Autodesk Inventor part; units mm, degrees
ref_plane "YZ Plane" through (0, 0, 0) normal (1, 0, 0) x (0, 1, 0)
ref_plane "XZ Plane" through (0, 0, 0) normal (0, 1, 0) x (-1, 0, 0)
ref_plane "XY Plane" through (0, 0, 0) normal (0, 0, 1) x (1, 0, 0)
sketch "Esboço1" plane through (0, 0, 0) normal (0, 0, 1) x (1, 0, 0)
  circle A0 centre (28.2, 9.3) radius 5.5
  line L0 (-31.3, -7.5) -> (33.7, -7.5) construction
  line L1 (33.7, -7.5) -> (33.7, 14.8) construction
  line L2 (33.7, 14.8) -> (-31.3, 14.8) construction
  line L3 (-31.3, 14.8) -> (-31.3, -7.5) construction
  circle A1 centre (10.85, -0.05) radius 5.5
  line L4 (-14.7338, -7.5) -> (-8.5113, -1.2775)
  line L5 (-31.3, -7.5) -> (-14.7338, -7.5)
  line L6 (-8.5113, -1.2775) -> (5.4887, -1.2775)
  line L7 (-31.3, -7.5) -> (-31.3, 0.8)
  line L8 (-31.3, 0.8) -> (-1.3563, 8.8234)
  line L9 (-1.3563, 8.8234) -> (3.6437, 8.8234)
  line L10 (3.6437, 8.8234) -> (26.4006, 14.4973)
  line L11 (14.415, 4.1381) -> (14.415, 6.5881)
  line L12 (14.415, 6.5881) -> (23.415, 6.5881)
  line L13 (-26.4266, -1) -> (-26.4266, -4.5)
  line L14 (-26.4266, -4.5) -> (-15.9765, -4.5)
  line L15 (-26.4266, -1) -> (-1.3377, 5.7225)
  line L16 (-15.9765, -4.5) -> (-9.7539, 1.7225)
  line L17 (-9.7539, 1.7225) -> (1.1623, 1.7225)
  line L18 (1.1623, 1.7225) -> (1.1623, 5.7225)
  line L19 (1.1623, 5.7225) -> (-1.3377, 5.7225)
  point P0 (0, 0)
  dimension "d4" = 11
  dimension "d5" = 28.2
  dimension "d6" = 9.3
  dimension "d7" = 65
  dimension "d8" = 22.3
  dimension "d9" = 65
  dimension "d10" = 9.35
  dimension "d11" = 17.35
  dimension "d12" = 8.8
  dimension "d14" = 135
  dimension "d15" = 14
  dimension "d16" = 8.3
  dimension "d17" = 31
  dimension "d18" = 105
  dimension "d19" = 5
  dimension "d20" = 14
  dimension "d21" = 2.45
  dimension "d22" = 9
  dimension "d23" = 3
  dimension "d24" = 3
  dimension "d25" = 3.5
  dimension "d26" = 3
  dimension "d27" = 3
  dimension "d28" = 4
  dimension "d29" = 2.5
extrude "Extrusão1" add sketch "Esboço1" along normal blind 2.2 contours A0 L12 L11 A1 L6 L4 L5 L7 L8 L9 L10
extrude "Extrusão2" add sketch "Esboço1" against normal blind 6.6 contours A1
extrude "Extrusão3" add sketch "Esboço1" along normal blind 2.2 contours A0
sketch "Esboço2" plane through (0, 0, 0) normal (0, 0, 1) x (1, 0, 0)
  arc A0 (5.4887, -1.2775) -> (14.415, 4.1381) centre (10.85, -0.05) ccw
  point P0 (0, 0)
hole "Furo1" at (10.85, -0.05, 0) direction (0, 0, -1) diameter 3.5 end through all
sketch "Esboço3" plane through (0, 0, 2.2) normal (0, 0, 1) x (1, 0, 0)
  arc A0 (23.415, 6.5881) -> (26.4006, 14.4973) centre (28.2, 9.3) ccw
  point P0 (0, 0)
hole "Furo2" at (28.2, 9.3, 2.2) direction (0, 0, -1) diameter 3.5 end through all countersink diameter 7 countersink angle 90
pattern_linear "Padrão retangular3" count 2 spacing 8.8 along (0, 0, -1) of "Extrusão1", "Extrusão3"
sketch "Esboço6" plane through (-14.7338, -7.5, -8.8) normal (0, 0, -1) x (-1, 0, 0)
  circle A0 centre (-42.9338, 16.8) radius 3.5
  line L0 (-41.1838, 13.7689) -> (-44.6838, 13.7689)
  line L1 (-44.6838, 13.7689) -> (-46.4338, 16.8)
  line L2 (-46.4338, 16.8) -> (-44.6838, 19.8311)
  line L3 (-44.6838, 19.8311) -> (-41.1838, 19.8311)
  line L4 (-41.1838, 19.8311) -> (-39.4338, 16.8)
  line L5 (-39.4338, 16.8) -> (-41.1838, 13.7689)
  point P0 (-14.7338, 7.5)
  point P1 (-42.9338, 16.8)
extrude "Extrusão6" cut sketch "Esboço6" along normal mid plane 4.4 contours L5 L0 L1 L2 L3 L4
sketch "Esboço4" plane through (0, 0, 0) normal (0, 0, -1) x (-1, 0, 0)
  line L0 (-26.4006, 14.4973) -> (-3.6437, 8.8234)
  line L1 (-26.4006, 14.4973) -> (-3.6437, 8.8234)
  line L2 (1.3563, 8.8234) -> (31.3, 0.8)
  line L3 (-3.6437, 8.8234) -> (1.3563, 8.8234)
  line L4 (1.3563, 8.8234) -> (31.3, 0.8)
  line L5 (31.3, 0.8) -> (31.3, -7.5)
  line L6 (31.3, -7.5) -> (14.7338, -7.5)
  line L7 (31.3, -7.5) -> (14.7338, -7.5)
  line L8 (14.7338, -7.5) -> (8.5113, -1.2775)
  line L9 (15.9765, -4.5) -> (9.7539, 1.7225)
  line L10 (8.5113, -1.2775) -> (-5.4887, -1.2775)
  arc A0 (-5.4887, -1.2775) -> (-14.415, 4.1381) centre (-10.85, -0.05) ccw
  arc A1 (-14.415, 4.1381) -> (-5.4887, -1.2775) centre (-10.85, -0.05) ccw
  line L11 (-14.415, 4.1381) -> (-14.415, 6.5881)
  line L12 (-14.415, 4.1381) -> (-14.415, 6.5881)
  line L13 (-14.415, 6.5881) -> (-23.415, 6.5881)
  line L14 (-14.415, 6.5881) -> (-23.415, 6.5881)
  arc A2 (-26.4006, 14.4973) -> (-23.415, 6.5881) centre (-28.2, 9.3) ccw construction
  arc A3 (-26.4006, 14.4973) -> (-23.415, 6.5881) centre (-28.2, 9.3) ccw
  arc A4 (-23.415, 6.5881) -> (-26.4006, 14.4973) centre (-28.2, 9.3) ccw
  line L15 (-1.1623, 5.7225) -> (1.3377, 5.7225)
  line L16 (-1.1623, 5.7225) -> (1.3377, 5.7225)
  line L17 (26.4266, -1) -> (1.3377, 5.7225)
  line L18 (1.3377, 5.7225) -> (26.4266, -1)
  line L19 (26.4266, -1) -> (26.4266, -4.5)
  line L20 (15.9765, -4.5) -> (26.4266, -4.5)
  line L21 (26.4266, -4.5) -> (15.9765, -4.5)
  line L22 (15.9765, -4.5) -> (9.7539, 1.7225)
  line L23 (9.7539, 1.7225) -> (-1.1623, 1.7225)
  line L24 (-1.1623, 1.7225) -> (-1.1623, 5.7225)
  point P0 (0, 0)
  point P1 (-5.4887, -1.2775)
extrude "Extrusão7" add sketch "Esboço4" along normal blind 6.6 contours L0 L3 L2 L5 L6 L8 L10 A0 L11 L13 A4
properties part number "Pinza_0002_001" material "Borracha"
Check sheet for the modelled part. Datum: model origin and axes. Units: mm. A direction names the side the tool comes from. Round coordinates to 2 decimals unless told otherwise and drop trailing zeros. Order: outer loops, then holes, each group sorted by start corner. A loop starts at its lowest first (then second) coordinate and runs counter-clockwise, first axis right, second up.
(1) Draft check along X on faces 6 (the flat face through (25.56, 7.81, -7.68)), 7 (the flat face through (1, 8.823, -3)), 8 (the flat face through (-16.119, 4.868, -3.223)), 9 (the flat face through (25.59, 10.84, -7.68)). Enter one of: pulls with the +X half, pulls with the -X half, needs draft (parallel to the pull), parting line crosses it, or undercut.
(2) Cross-section at D-D, the plane z = -5. State how many separate pieces and enclosed holes the cut face has, and give its area (3 significant figures).
(3) Access from +Z, -Z, +X, -X, +Y, -Y to the whole of each face (thin tool, end or side, straight path). Record for faces 1 (the flat face through (0, 5.722, -3)), 2 (the flat face through (1, 6, -8.8)), 3 (the flat face through (-31.3, -3, -3)), 4 (the cylindrical face through (7.915, 4.602, 1.085)), 5 (the flat face through (30.84, 10.79, -7.68)).
(4) Go/stop test with flat-tipped pins: P1, Ø4, axis at y = -3, z = -3.5, coming from the +X side; P2, Ø0.7, axis at x = 28, z = -7.5, coming from the -Y side; P3, Ø2.5, axis at x = 1, z = -1.5, coming from the +Y side; P4, Ø12, axis at x = 8.5, y = 0.5, coming from the +Z side. Record where each tip stops, or that it passes through.
(5) Cross-section at B-B, the plane x = -24. Enter the section's corners in (y, z), and give its area (3 significant figures).
(6) Cross-section at A-A, the plane x = 28.2. Enter the section's corners in (y, z).
(7) Cross-section at C-C, the plane y = -3.25. Enter the section's corners in (x, z).
(8) Scan lines: probe 1 along Z at (x, y) = (30, 5.25); probe 2 along Y at (x, z) = (28.2, 0.35); probe 3 along X at (y, z) = (-1.5, -3). Record each from-to range of solid material in increasing order.
Check sheet entries:
1. face 6: undercut
1. face 7: needs draft
1. face 8: pulls with the -X half
1. face 9: undercut
2. separate pieces: 1
2. enclosed holes: 2
2. area: 454 mm2
3. face 1: +Z, -Z
3. face 2: -Z, +X, -X, +Y, -Y
3. face 3: +Z, -Z, -X, +Y, -Y
3. face 4: +Z
3. face 5: -Z
4. P1: stops at x = 16.27
4. P2: stops at y = 3.8
4. P3: stops at y = 8.82
4. P4: stops at z = 2.2
5. outline: (-7.5, -8.8) - (-4.5, -8.8) - (-4.5, 2.2) - (-7.5, 2.2) - close; (-0.35, -8.8) - (2.76, -8.8) - (2.76, 2.2) - (-0.35, 2.2) - close
5. area: 67.2 mm2
6. outline: (3.8, -8.8) - (6.27, -8.8) - (6.27, -6.6) - (3.8, -6.6) - close; (3.8, 0) - (7.55, 0) - (7.55, 0.45) - (5.8, 2.2) - (3.8, 2.2) - close; (11.05, 0) - (14.8, 0) - (14.8, 2.2) - (12.8, 2.2) - (11.05, 0.45) - close; (12.33, -8.8) - (14.8, -8.8) - (14.8, -6.6) - (12.33, -6.6) - close
7. outline: (-31.3, -8.8) - (-26.43, -8.8) - (-26.43, 2.2) - (-31.3, 2.2) - close; (-14.73, -8.8) - (-10.48, -8.8) - (-10.48, 2.2) - (-14.73, 2.2) - close; (6.38, -6.6) - (15.32, -6.6) - (15.32, 0) - (6.38, 0) - close
8. probe 1: z = -8.8 to -6.6, 0 to 2.2
8. probe 2: y = 3.8 to 7.55, 11.05 to 14.8
8. probe 3: x = -31.3 to -26.43, -12.98 to -8.73, 5.54 to 9.87, 11.83 to 16.16
